```python
from build123d import *

# Parameters (mm, degrees)
SKETCH3_R          = 1.25
CUT_EXTRUDE1_DEPTH = 15.477914214


with BuildPart() as part:
    # Sketch2 → Revolve1 (revolve)
    with BuildSketch(Plane.XY, mode=Mode.PRIVATE) as revolve1_sk:
        Polygon((1.75, 0), (10, 0), (10, -0.6), (4.55, -0.6), (4.55, -3.1), (2.75, -3.1), (2.75, -0.6), (1.75, -0.6), align=None)
    revolve(revolve1_sk.sketch.rotate(Axis((0, 0, 0), (0, -1, 0)), 180), axis=Axis((0, 0, 0), (0, -1, 0)))

    # Sketch3 → Cut-Extrude1 (cut, through all)
    with BuildSketch(Plane(origin=(0, 0, 0), x_dir=(1, 0, 0), z_dir=(0, 1, 0))):
        with Locations(Location((0, 7, 0), (0, 0, 180))):
            Circle(SKETCH3_R)
        with Locations(Location((7, 0, 0), (0, 0, 180))):
            Circle(SKETCH3_R)
        with Locations(Location((0, -7, 0), (0, 0, 180))):
            Circle(SKETCH3_R)
        with Locations(Location((-7, 0, 0), (0, 0, 180))):
            Circle(SKETCH3_R)
    extrude(amount=-CUT_EXTRUDE1_DEPTH, mode=Mode.SUBTRACT)


solid = part.part
```
The listing builds one solid part. Answer for the finished solid, in the listing's coordinates (mm). A direction names the side the tool comes from. Give positions to 0.01 mm unless a question says otherwise; leave off trailing zeros. Order: outer loops, then holes, each group sorted by start corner. A loop starts at its lowest first (then second) coordinate and runs counter-clockwise, first axis right, second up. Notation, with made-up numbers: (-21.5, 75) - (12.5, 75) arc R18 cw to (12.5, 99) - close; hole circle Ø5 at (35.25, 39). An arc over 180 degrees is marked (long way). Answer in a Markdown table with one row per item. Add a question column.
Q1. The part is cut by section B-B (z = 0). Determine the outline of the cut face in (x, y).
Q2. Find the intervals of material crossed by line 1 along Z through (x, y) = (0, -0.4); line 2 along Y through (x, z) = (-6.5, 3.25); line 3 along Z through (x, y) = (1.5, -1.25), in increasing order. Write a range as [from, to].
Q3. The part is cut by section A-A (x = 0). Determine the outline of the cut face in (y, z), then the cut area to 3 significant figures.
Q4. The part is cut by section D-D (z = -7). Determine the outline of the cut face in (x, y), then the cut area to 3 significant figures.
Q5. Given P1, Ø3, axis at x = -7, z = 0, coming from the -Y side; P2, Ø1.5, axis at x = -5, y = -1, coming from the +Z side; P3, Ø1.5, axis at y = -1, z = 1, coming from the +X side, each flat-ended and moving along its own axis, determine where each tip first touches the part or whether it passes through.
Q6. Which of the six approach directions +Z, -Z, +X, -X, +Y, -Y give full straight-line access (tool end or side, diameter ignored) to faces 4 (the cylindrical face through (0.596, -1.832, 2.685)), 5 (the flat face through (0, -3.1, 3))?
Q7. For a pull along Z with two mould halves and no side action, classify faces 1 (the flat face through (0, 0, 2)), 2 (the cylindrical face through (0.27, -0.3, 5.78)), 3 (the cylindrical face through (3.61, -1.87, 2.77)) as released by +Z, released by -Z, zero draft, split by the parting line, or undercut.
Q8. The part is cut by section C-C (x = 8). Determine the outline of the cut face in (y, z).
Determined:
| question | item | result |
|---|---|---|
| 1 | outline | (-10, -0.6) - (-8.25, -0.6) - (-8.25, 0) - (-10, 0) - close; (-5.75, -0.6) - (-4.55, -0.6) - (-4.55, -3.1) - (-2.75, -3.1) - (-2.75, -0.6) - (-1.75, -0.6) - (-1.75, 0) - (-5.75, 0) - close; (1.75, -0.6) - (2.75, -0.6) - (2.75, -3.1) - (4.55, -3.1) - (4.55, -0.6) - (5.75, -0.6) - (5.75, 0) - (1.75, 0) - close; (8.25, -0.6) - (10, -0.6) - (10, 0) - (8.25, 0) - close |
| 2 | line 1 | z = [-10, -8.25], [-5.75, -1.75], [1.75, 5.75], [8.25, 10] |
| 2 | line 2 | y = [-0.6, 0] |
| 2 | line 3 | z = [-4.3, -2.3], [2.3, 4.3] |
| 3 | outline | (-3.1, -4.55) - (-0.6, -4.55) - (-0.6, -5.75) - (0, -5.75) - (0, -1.75) - (-0.6, -1.75) - (-0.6, -2.75) - (-3.1, -2.75) - close; (-3.1, 2.75) - (-0.6, 2.75) - (-0.6, 1.75) - (0, 1.75) - (0, 5.75) - (-0.6, 5.75) - (-0.6, 4.55) - (-3.1, 4.55) - close; (-0.6, -10) - (0, -10) - (0, -8.25) - (-0.6, -8.25) - close; (-0.6, 8.25) - (0, 8.25) - (0, 10) - (-0.6, 10) - close |
| 3 | area | 15.9 mm² |
| 4 | outline | (-7.14, -0.6) - (-1.25, -0.6) - (-1.25, 0) - (-7.14, 0) - close; (1.25, -0.6) - (7.14, -0.6) - (7.14, 0) - (1.25, 0) - close |
| 4 | area | 7.07 mm² |
| 5 | P1 | stops at y = -0.6 |
| 5 | P2 | stops at z = 9 |
| 5 | P3 | stops at x = 9.99 |
| 6 | face 4 | -Y |
| 6 | face 5 | +Z, -Z, +X, -X, -Y |
| 7 | face 1 | zero draft |
| 7 | face 2 | undercut |
| 7 | face 3 | split by the parting line |
| 8 | outline | (-0.6, -6) - (0, -6) - (0, -0.75) - (-0.6, -0.75) - close; (-0.6, 0.75) - (0, 0.75) - (0, 6) - (-0.6, 6) - close |
